Could you check a few things on this model? Use its own coordinates, in mm. A direction names the side the tool comes from. Give positions to 0.01 mm unless a question says otherwise; leave off trailing zeros. One line per question, with ' | ' between items.
from build123d import *

# Parameters (mm, degrees)
F0_W     = 90
F0_H     = 55
F1_DEPTH = 30
F3_DEPTH = 90
F5_DEPTH = 60


with BuildPart() as f1:
    # F0 (on Top) → F1 (new body)
    with BuildSketch(Plane.XY):
        with Locations((45, -27.5)):
            Rectangle(F0_W, F0_H)
    extrude(amount=F1_DEPTH)

    # F2 (on face) → F3 (cut)
    with BuildSketch(Plane.XZ.offset(55)):
        Polygon((3.3461908971, 0), (0, 3.2115780663), (0, 0), align=None)
        Polygon((6.4285714286, 3.2115780663), (3.3461908971, 0), (9.7747623256, 0), align=None)
        Polygon((12.8571428571, 3.2115780663), (9.7747623256, 0), (16.2033337542, 0), align=None)
        Polygon((19.2857142857, 3.2115780663), (16.2033337542, 0), (22.6319051828, 0), align=None)
        Polygon((25.7142857143, 3.2115780663), (22.6319051828, 0), (29.0604766113, 0), align=None)
        Polygon((32.1428571429, 3.2115780663), (29.0604766113, 0), (35.4890480399, 0), align=None)
        Polygon((38.5714285714, 3.2115780663), (35.4890480399, 0), (41.9176194685, 0), align=None)
        Polygon((45, 3.2115780663), (41.9176194685, 0), (48.3461908971, 0), align=None)
        Polygon((51.4285714286, 3.2115780663), (48.3461908971, 0), (54.7747623256, 0), align=None)
        Polygon((54.7747623256, 0), (61.2033337542, 0), (57.8571428571, 3.2115780663), align=None)
        Polygon((61.2033337542, 0), (67.6319051828, 0), (64.2857142857, 3.2115780663), align=None)
        Polygon((67.6319051828, 0), (74.0604766113, 0), (70.7142857143, 3.2115780663), align=None)
        Polygon((74.0604766113, 0), (80.4890480399, 0), (77.1428571429, 3.2115780663), align=None)
        Polygon((80.4890480399, 0), (86.9176194685, 0), (83.5714285714, 3.2115780663), align=None)
        Polygon((90, 0), (90, 3.2115780663), (86.9176194685, 0), align=None)
    extrude(amount=-F3_DEPTH, mode=Mode.SUBTRACT)

    # F4 (on face) → F5 (cut)
    with BuildSketch(Plane.XZ.offset(55)):
        Polygon((0, 1.6057890331), (0, 0), (3.3461908971, 0), (1.6730954485, 1.6057890331), align=None)
        Polygon((90, 1.6057890331), (88.4588097342, 1.6057890331), (86.9176194685, 0), (90, 0), align=None)
        Polygon((4.8873811628, 1.6057890331), (3.3461908971, 0), (9.7747623256, 0), (8.1016668771, 1.6057890331), align=None)
        Polygon((11.3159525914, 1.6057890331), (9.7747623256, 0), (16.2033337542, 0), (14.5302383057, 1.6057890331), align=None)
        Polygon((24.1730954485, 1.6057890331), (22.6319051828, 0), (29.0604766113, 0), (27.3873811628, 1.6057890331), align=None)
        Polygon((30.6016668771, 1.6057890331), (29.0604766113, 0), (35.4890480399, 0), (33.8159525914, 1.6057890331), align=None)
        Polygon((37.0302383057, 1.6057890331), (35.4890480399, 0), (41.9176194685, 0), (40.24452402, 1.6057890331), align=None)
        Polygon((43.4588097342, 1.6057890331), (41.9176194685, 0), (48.3461908971, 0), (46.6730954485, 1.6057890331), align=None)
        Polygon((49.8873811628, 1.6057890331), (48.3461908971, 0), (54.7747623256, 0), (53.1016668771, 1.6057890331), align=None)
        Polygon((56.3159525914, 1.6057890331), (54.7747623256, 0), (61.2033337542, 0), (59.5302383057, 1.6057890331), align=None)
        Polygon((62.74452402, 1.6057890331), (61.2033337542, 0), (67.6319051828, 0), (65.9588097342, 1.6057890331), align=None)
        Polygon((67.6319051828, 0), (74.0604766113, 0), (72.3873811628, 1.6057890331), (69.1730954485, 1.6057890331), align=None)
        Polygon((74.0604766113, 0), (80.4890480399, 0), (78.8159525914, 1.6057890331), (75.6016668771, 1.6057890331), align=None)
        Polygon((86.9176194685, 0), (85.24452402, 1.6057890331), (82.0302383057, 1.6057890331), (80.4890480399, 0), align=None)
        Polygon((1.6730954485, 1.6057890331), (3.3461908971, 0), (4.8873811628, 1.6057890331), align=None)
        Polygon((8.1016668771, 1.6057890331), (9.7747623256, 0), (11.3159525914, 1.6057890331), align=None)
        Polygon((14.5302383057, 1.6057890331), (16.2033337542, 0), (17.74452402, 1.6057890331), align=None)
        Polygon((20.9588097342, 1.6057890331), (22.6319051828, 0), (24.1730954485, 1.6057890331), align=None)
        Polygon((27.3873811628, 1.6057890331), (29.0604766113, 0), (30.6016668771, 1.6057890331), align=None)
        Polygon((33.8159525914, 1.6057890331), (35.4890480399, 0), (37.0302383057, 1.6057890331), align=None)
        Polygon((40.24452402, 1.6057890331), (41.9176194685, 0), (43.4588097342, 1.6057890331), align=None)
        Polygon((46.6730954485, 1.6057890331), (48.3461908971, 0), (49.8873811628, 1.6057890331), align=None)
        Polygon((53.1016668771, 1.6057890331), (54.7747623256, 0), (56.3159525914, 1.6057890331), align=None)
        Polygon((59.5302383057, 1.6057890331), (61.2033337542, 0), (62.74452402, 1.6057890331), align=None)
        Polygon((65.9588097342, 1.6057890331), (67.6319051828, 0), (69.1730954485, 1.6057890331), align=None)
        Polygon((72.3873811628, 1.6057890331), (74.0604766113, 0), (75.6016668771, 1.6057890331), align=None)
        Polygon((80.4890480399, 0), (82.0302383057, 1.6057890331), (78.8159525914, 1.6057890331), align=None)
        Polygon((86.9176194685, 0), (88.4588097342, 1.6057890331), (85.24452402, 1.6057890331), align=None)
    extrude(amount=-F5_DEPTH, mode=Mode.SUBTRACT)


solid = f1.part
Q1. If I drill on line 1 along Z through (x, y) = (18, -4.5); line 2 along Z through (x, y) = (14.5, -25.5), over which ranges is the centre line in solid material (lowest first)?
Answer below:
line 1: z = 1.87 to 30 | line 2: z = 1.63 to 30
Q2. If we mould it in two halves opening along X, with no side actions, what happens to faces 3 (the flat face through (44, -55, 16)), 4 (the flat face through (0, -28, 16)), 5 (the flat face through (13.7, -27.9, 2.4))? For each: +X half, -X half, draft (parallel to the pull), parting line (faces both ways), or undercut.
Answer below:
face 3: draft | face 4: -X half | face 5: undercut
Q3. On a 3-axis mill with a long thin cutter (end or side, diameter ignored), from which of +Z, -Z, +X, -X, +Y, -Y can I reach the whole of each face in a straight line? I mean faces 1 (the flat face through (32.99, -27.88, 2.4)), 2 (the flat face through (44, -27, 30)). Say none if no direction works.
Answer below:
face 1: -Z, +Y, -Y | face 2: +Z, +X, -X, +Y, -Y
